Can you work these out from the model? Positions are in its coordinate system, mm. A direction names the side the tool comes from. Give positions to 0.01 mm unless a question says otherwise; leave off trailing zeros. Loops run counter-clockwise (first coordinate to the right, second up) from the corner with the lowest first, then second, coordinate; pieces in that order, holes last.
from build123d import *

# Parameters (mm, degrees)
BOSS_EXTRUDE1_DEPTH     = 76.2
SKETCH3_W               = 22.86
SKETCH3_H               = 68.58
CUT_EXTRUDE1_DEPTH      = 76.2
SKETCH4_W               = 27.94
SKETCH4_H               = 13.05965896
BOSS_EXTRUDE2_DEPTH     = 0.762
CUT_EXTRUDE2_DEPTH      = 99.822
SKETCH7_W               = 27.94
SKETCH7_H               = 13.05965896
BOSS_EXTRUDE3_DEPTH     = 1.27
SKETCH8_R               = 3.81
BOSS_EXTRUDE4_DEPTH     = 12.7
CUT_EXTRUDE3_DEPTH      = 116.55549125
CUT_EXTRUDE3_DEPTH_BACK = 116.55549125
SKETCH10_W              = 1.211973452
SKETCH10_H              = 6.241961148


with BuildPart() as part:
    # Sketch2 → Boss-Extrude1 (new body)
    with BuildSketch(Plane.XY):
        Polygon((-1.796051224, 1.796051224), (-5.388153673, 5.388153673), (-5.388153673, 10.468153673), (5.388153673, 10.468153673), (5.388153673, 5.388153673), (1.796051224, 1.796051224), (1.796051224, 0), (5.388153673, 0), (7.928153673, 0), (7.928153673, 10.468153673), (19.358153673, 10.468153673), (31.75, 10.468153673), (36.83, 10.468153673), (36.83, -2.591505287), (31.75, -2.591505287), (-31.75, -2.591505287), (-36.83, -2.591505287), (-36.83, 10.468153673), (-31.75, 10.468153673), (-19.358153673, 10.468153673), (-7.928153673, 10.468153673), (-7.928153673, 0), (-1.796051224, 0), align=None)
    extrude(amount=BOSS_EXTRUDE1_DEPTH)

    # Sketch3 → Cut-Extrude1 (cut)
    with BuildSketch(Plane(origin=(0, 10.468153673, 0), x_dir=(1, 0, 0), z_dir=(0, 1, 0))):
        with Locations((-25.4, -41.91)):
            Rectangle(SKETCH3_W, SKETCH3_H)
        with Locations((25.4, -41.91)):
            Rectangle(SKETCH3_W, SKETCH3_H)
    extrude(amount=-CUT_EXTRUDE1_DEPTH, mode=Mode.SUBTRACT)

    # Sketch4 → Boss-Extrude2 (add)
    with BuildSketch(Plane.XY.offset(76.2)):
        with Locations((0, 3.938324193)):
            Rectangle(SKETCH4_W, SKETCH4_H)
    extrude(amount=BOSS_EXTRUDE2_DEPTH)

    # Sketch5 → Cut-Extrude2 (cut)
    with BuildSketch(Plane.XY.offset(76.962)):
        Polygon((1.329001146, -2.591505287), (1.329001146, 0.714117771), (2.850653855, 0.714117771), (2.850653855, 1.492637762), (1.329001146, 1.492637762), (0, 1.492637762), (0, 0.714117771), (0, -2.591505287), align=None)
    extrude(amount=-CUT_EXTRUDE2_DEPTH, mode=Mode.SUBTRACT)

    # Sketch7 → Boss-Extrude3 (add)
    with BuildSketch(Plane.XY.offset(76.962)):
        with Locations((0, 3.938324193)):
            Rectangle(SKETCH7_W, SKETCH7_H)
    extrude(amount=BOSS_EXTRUDE3_DEPTH)

    # Sketch8 → Boss-Extrude4 (add)
    with BuildSketch(Plane.XZ.offset(2.591505287)):
        with Locations(Location((-31.115, 3.81, 0), (0, 0, 270))):
            Circle(SKETCH8_R)
        with Locations(Location((31.115, 3.81, 0), (0, 0, 270))):
            Circle(SKETCH8_R)
    extrude(amount=BOSS_EXTRUDE4_DEPTH)

    # Sketch10 → Cut-Extrude3 (cut, two sides: drawn at the far end of the back side and taken through both)
    with BuildSketch(Plane.ZY.offset(46.83).offset(-CUT_EXTRUDE3_DEPTH_BACK)):
        with Locations((0.605986726, -9.213101257)):
            Rectangle(SKETCH10_W, SKETCH10_H)
    extrude(amount=CUT_EXTRUDE3_DEPTH + CUT_EXTRUDE3_DEPTH_BACK, mode=Mode.SUBTRACT)


solid = part.part
(1) Suppose I cut it at D-D on z = 57.5. List the corners of the cut face in (x, y) for me.
Returned:
outline: (-13.97, -2.59) - (0, -2.59) - (0, 1.49) - (1.8, 1.49) - (1.8, 1.8) - (5.39, 5.39) - (5.39, 10.47) - (-5.39, 10.47) - (-5.39, 5.39) - (-1.8, 1.8) - (-1.8, 0) - (-7.93, 0) - (-7.93, 10.47) - (-13.97, 10.47) - close; (1.33, -2.59) - (13.97, -2.59) - (13.97, 10.47) - (7.93, 10.47) - (7.93, 0) - (1.8, 0) - (1.8, 0.71) - (1.33, 0.71) - close
(2) Suppose I cut it at C-C on y = -8. List the corners of the cut face in (x, z) for me (3 decimals).
Returned:
outline: (-33.902, 1.212) - (-28.328, 1.212) arc R3.81 ccw (long way) to start; (28.328, 1.212) - (33.902, 1.212) arc R3.81 ccw (long way) to start
(3) Suppose I cut it at B-B on y = 7. List the corners of the cut face in (x, z) for me, plus the area to 3 significant figures.
Returned:
outline: (-36.83, 0) - (-7.93, 0) - (-7.93, 76.2) - (-5.39, 76.2) - (-5.39, 0) - (5.39, 0) - (5.39, 76.2) - (7.93, 76.2) - (7.93, 0) - (36.83, 0) - (36.83, 7.62) - (13.97, 7.62) - (13.97, 78.23) - (-13.97, 78.23) - (-13.97, 7.62) - (-36.83, 7.62) - close
area: 2,150 mm2
(4) Please list where these lines run through material, in increasing order: probe 1 along X at (y, z) = (7, 17); probe 2 along X at (y, z) = (-2.5, 51.5); probe 3 along Y at (x, z) = (5.5, 67.5).
Returned:
probe 1: x = -13.97 to -7.93, -5.39 to 5.39, 7.93 to 13.97
probe 2: x = -13.97 to 0, 1.33 to 13.97
probe 3: y = -2.59 to 0
(5) Thinking about a two-plate mould opening in Y: for faces 1 (the flat face through (4, 4, 38)), 2 (the flat face through (23, 4, 0)), 3 (the flat face through (-31, -15.292, 4)), which applies, pulls with the +Y half, pulls with the -Y half, needs draft (parallel to the pull), parting line crosses it, or undercut?
Returned:
face 1: undercut
face 2: needs draft
face 3: pulls with the -Y half
(6) Which directions (+Z, -Z, +X, -X, +Y, -Y) give clear straight access to the entire face, cutting with the end or side of a thin tool? Please do faces 4 (the flat face through (0, -1, 39)), 5 (the flat face through (35.2, -2.592, 3.8)), 6 (the flat face through (-5.388, 8, 38)), 7 (the flat face through (13.97, 4, 42)), 8 (the flat face through (31, -9, 1.212)).
Returned:
face 4: -Z, -Y
face 5: +X, -Y
face 6: -Z, +Y
face 7: +Z, +X, +Y, -Y
face 8: -Z, +X, -X
(7) Will these pins go through, and if not, where does the flat tip stop? P1, Ø10, axis at y = 6.5, z = 29.5, coming from the +X side; P2, Ø2, axis at x = 17.5, y = 2, coming from the +Z side; P3, Ø6, axis at x = -18, y = 3.5, coming from the -Z side; P4, Ø1.4, axis at y = 0.5, z = 20.5, coming from the -X side.
Returned:
P1: stops at x = 13.97
P2: stops at z = 7.62
P3: stops at z = 0
P4: stops at x = -13.97
